Part model, mm, in its own coordinate system. Give positions to 0.01 mm unless a question says otherwise; leave off trailing zeros. Order: outer loops, then holes, each group sorted by start corner. A loop starts at its lowest first (then second) coordinate and runs counter-clockwise, first axis right, second up. Notation, with made-up numbers: (74, -17) - (81, -17) arc R13 ccw to (81, -8) - close; hole circle Ø4 at (-16.5, 67). An arc over 180 degrees is marked (long way). One line per item, written item: value.
```python
from build123d import *

# Parameters (mm, degrees)
ESBO_O1_R                = 18.5
ESBO_O1_R_2              = 4.5
ESBO_O1_R_3              = 5
ESBO_O1_R_4              = 1.8
ESBO_O1_R_5              = 3
ESBO_O1_R_6              = 1.75
RESSALTO_EXTRUS_O1_DEPTH = 6


with BuildPart() as part:
    # Esboço1 → Ressalto-extrusão1 (new body)
    with BuildSketch(Plane.XY):
        with BuildLine():
            Line((100, -25), (100, -21))
            Line((100, -21), (96.7, -21))
            Line((96.7, -21), (96.7, -17))
            Line((96.7, -17), (100, -17))
            Line((100, -17), (100, -16))
            Line((100, -16), (97.8, -16))
            Line((97.8, -16), (97.8, -13))
            Line((97.8, -13), (96.7, -13))
            Line((96.7, -13), (96.7, -11))
            Line((96.7, -11), (93.3, -11))
            Line((93.3, -11), (93.3, -13))
            Line((93.3, -13), (92.2, -13))
            Line((92.2, -13), (92.2, -16))
            Line((92.2, -16), (90, -16))
            Line((90, -16), (90, -17))
            Line((90, -17), (93.3, -17))
            Line((93.3, -17), (93.3, -21))
            Line((93.3, -21), (90, -21))
            Line((90, -21), (90, -25))
            Line((90, -25), (-27.5, -25))
            Line((-27.5, -25), (-27.5, -21))
            Line((-27.5, -21), (-30.8, -21))
            Line((-30.8, -21), (-30.8, -17))
            Line((-30.8, -17), (-27.5, -17))
            Line((-27.5, -17), (-27.5, -16))
            Line((-27.5, -16), (-29.7, -16))
            Line((-29.7, -16), (-29.7, -13))
            Line((-29.7, -13), (-30.8, -13))
            Line((-30.8, -13), (-30.8, -11))
            Line((-30.8, -11), (-34.2, -11))
            Line((-34.2, -11), (-34.2, -13))
            Line((-34.2, -13), (-35.3, -13))
            Line((-35.3, -13), (-35.3, -16))
            Line((-35.3, -16), (-37.5, -16))
            Line((-37.5, -16), (-37.5, -17))
            Line((-37.5, -17), (-34.2, -17))
            Line((-34.2, -17), (-34.2, -21))
            Line((-34.2, -21), (-37.5, -21))
            Line((-37.5, -21), (-37.5, -25))
            Line((-37.5, -25), (-110, -25))
            ThreePointArc((-110, -25), (-117.071067812, -22.071067812), (-120, -15))
            Line((-120, -15), (-120, 15))
            ThreePointArc((-120, 15), (-117.071067812, 22.071067812), (-110, 25))
            Line((-110, 25), (110, 25))
            ThreePointArc((110, 25), (117.071067812, 22.071067812), (120, 15))
            Line((120, 15), (116, 15))
            Line((116, 15), (116, 11.7))
            Line((116, 11.7), (112, 11.7))
            Line((112, 11.7), (112, 15))
            Line((112, 15), (111, 15))
            Line((111, 15), (111, 12.8))
            Line((111, 12.8), (108, 12.8))
            Line((108, 12.8), (108, 11.7))
            Line((108, 11.7), (106, 11.7))
            Line((106, 11.7), (106, 8.3))
            Line((106, 8.3), (108, 8.3))
            Line((108, 8.3), (108, 7.2))
            Line((108, 7.2), (111, 7.2))
            Line((111, 7.2), (111, 5))
            Line((111, 5), (112, 5))
            Line((112, 5), (112, 8.3))
            Line((112, 8.3), (116, 8.3))
            Line((116, 8.3), (116, 5))
            Line((116, 5), (120, 5))
            Line((120, 5), (120, -15))
            ThreePointArc((120, -15), (117.071067812, -22.071067812), (110, -25))
            Line((110, -25), (100, -25))
        make_face()
        with Locations((-80, 0)):
            Circle(ESBO_O1_R, mode=Mode.SUBTRACT)
        with Locations((100, 0)):
            Circle(ESBO_O1_R_2, mode=Mode.SUBTRACT)
        with Locations((8, 0)):
            Circle(ESBO_O1_R_3, mode=Mode.SUBTRACT)
        with Locations((-108.81, 0)):
            Circle(ESBO_O1_R_2, mode=Mode.SUBTRACT)
        with Locations((-14.5, 0)):
            Circle(ESBO_O1_R_4, mode=Mode.SUBTRACT)
        with Locations((30.5, 0)):
            Circle(ESBO_O1_R_4, mode=Mode.SUBTRACT)
        with Locations((-29.5, 12.5)):
            Circle(ESBO_O1_R_5, mode=Mode.SUBTRACT)
        with Locations((45.5, 12.5)):
            Circle(ESBO_O1_R_5, mode=Mode.SUBTRACT)
        with Locations((-101.81, 14)):
            Circle(ESBO_O1_R_6, mode=Mode.SUBTRACT)
        with Locations((-101.81, -14)):
            Circle(ESBO_O1_R_6, mode=Mode.SUBTRACT)
    extrude(amount=RESSALTO_EXTRUS_O1_DEPTH)


solid = part.part
```
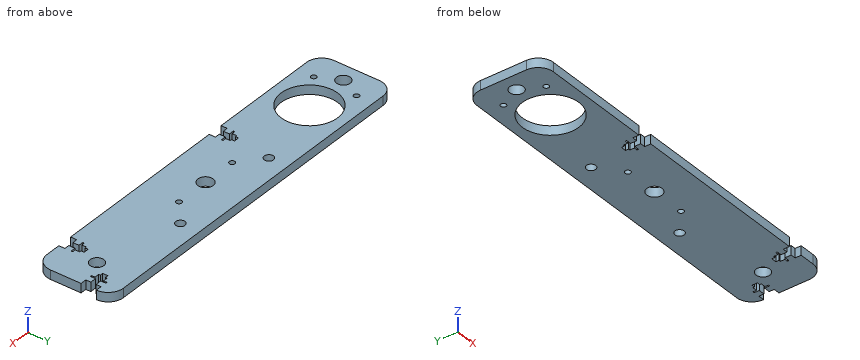
1) Cut at B-B, the plane z = 2.55. Give the number of separate pieces and of enclosed holes in the cut face, then the cut area to 3 significant figures.
Outcome:
separate pieces: 1
enclosed holes: 10
area: 10,300 mm^2
2) Pin check, flat tips, straight feed: pin 1 (2.5 mm diameter, centred on x = 94.5, z = 4, fed in from -Y); pin 2 (3.5 mm diameter, centred on x = -29.5, y = 12.5, fed in from +Z); pin 3 (3 mm diameter, centred on y = -23, z = 3.5, fed in from +X); pin 4 (1.1 mm diameter, centred on x = 111.5, z = 4, fed in from -Y). Stop position of each tip, or through.
Outcome:
pin 1: stops at y = -21
pin 2: passes through
pin 3: stops at x = 117.6
pin 4: stops at y = -24.95
3) Cut at A-A, the plane x = 8. Give the cut face in (y, z), then the cut area to 3 significant figures.
Outcome:
outline: (-25, 0) - (-5, 0) - (-5, 6) - (-25, 6) - close; (5, 0) - (25, 0) - (25, 6) - (5, 6) - close
area: 240 mm^2
4) Cut at C-C, the plane x = 45.5. Give the cut face in (y, z), then the cut area to 3 significant figures.
Outcome:
outline: (-25, 0) - (9.5, 0) - (9.5, 6) - (-25, 6) - close; (15.5, 0) - (25, 0) - (25, 6) - (15.5, 6) - close
area: 264 mm^2
5) Drill centre lines: line 1 along Y through (x, z) = (-35.5, 4.85); line 2 along Y through (x, z) = (-80, 2.25); line 3 along X through (y, z) = (-3, 4.9). Where is each one in solid material? Low to high. Write a range as from..to.
Outcome:
line 1: y = -21..-17, -16..25
line 2: y = -25..-18.5, 18.5..25
line 3: x = -120..-112.16, -105.46..-98.26, -61.74..4, 12..96.65, 103.35..120
